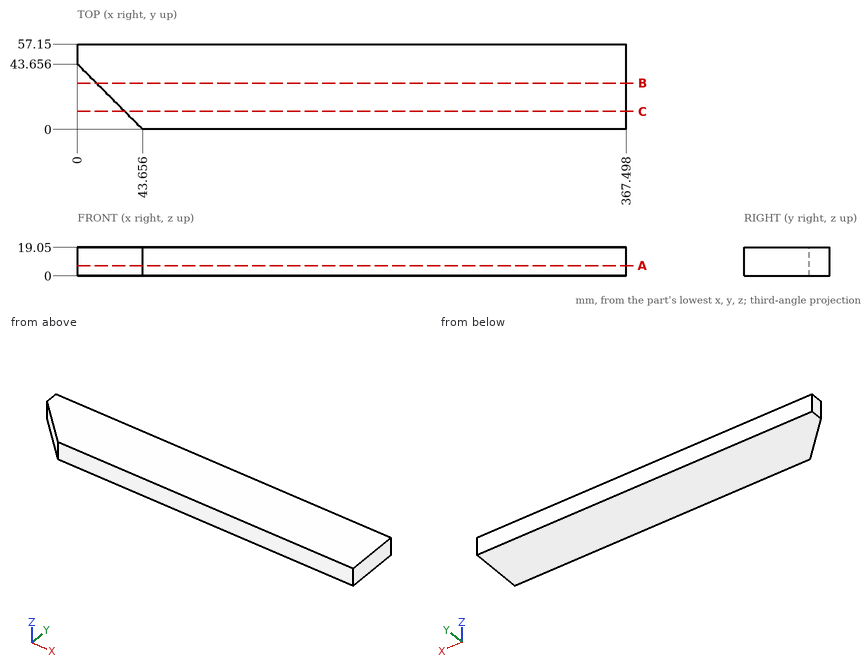
Input: dimensioned drawing with shaded views. Units: mm. Origin: part minimum x, y, z. Give positions to 0.01 mm unless a question says otherwise; leave off trailing zeros. Loops run counter-clockwise (first coordinate to the right, second up) from the corner with the lowest first, then second, coordinate; pieces in that order, holes last. Notation, with made-up numbers: (23, -38.5) -> (63, -38.5) arc R7 cw to (63, -32.5) -> close; hole circle Ø3 at (-6.75, -31). An arc over 180 degrees is marked (long way). Use a Markdown table: item, result.
Q1. Ray query, probe 1 along X at (y, z) = (30.5, 6.75) (1 decimal); probe 2 along X at (y, z) = (20.5, 10.5) (1 decimal). Return the intervals inside material, ascending. Write a range as from..to.
Entries:
| item | result |
|---|---|
| probe 1 | x = 13.2..367.5 |
| probe 2 | x = 23.2..367.5 |
Q2. Section query C-C, the plane y = 12. Return the cut outline in (x, z), plus the area to 3 significant figures.
Entries:
| item | result |
|---|---|
| outline | (31.66, 0) -> (367.5, 0) -> (367.5, 19.05) -> (31.66, 19.05) -> close |
| area | 6,400 mm² |
Q3. Section query B-B, the plane y = 31. Return the cut outline in (x, z).
Entries:
| item | result |
|---|---|
| outline | (12.66, 0) -> (367.5, 0) -> (367.5, 19.05) -> (12.66, 19.05) -> close |
Q4. Section query A-A, the plane z = 6.75. Return the cut outline in (x, y), plus the area to 4 significant figures.
Entries:
| item | result |
|---|---|
| outline | (0, 43.66) -> (43.66, 0) -> (367.5, 0) -> (367.5, 57.15) -> (0, 57.15) -> close |
| area | 20,050 mm² |
